```python
from build123d import *

# Parameters (mm, degrees)
SKETCH1_R           = 20
BOSS_EXTRUDE1_DEPTH = 5
SKETCH3_R           = 3
BOSS_EXTRUDE2_DEPTH = 11
CUT_EXTRUDE1_DEPTH  = 6


with BuildPart() as part:
    # Sketch1 → Boss-Extrude1 (new body)
    with BuildSketch(Plane.XY):
        Circle(SKETCH1_R)
    extrude(amount=BOSS_EXTRUDE1_DEPTH)

    # Sketch3 → Boss-Extrude2 (add)
    with BuildSketch(Plane.XY.offset(5)):
        with Locations((-15, 0)):
            Circle(SKETCH3_R)
    extrude(amount=BOSS_EXTRUDE2_DEPTH)

    # Sketch5 → Cut-Extrude1 (cut, through all)
    with BuildSketch(Plane.XY.offset(5)):
        with BuildLine():
            Line((5.656854249, 2), (7.5, 2))
            Line((7.5, 2), (7.5, -2))
            Line((7.5, -2), (5.656854249, -2))
            ThreePointArc((5.656854249, -2), (-6, 0), (5.656854249, 2))
        make_face()
    extrude(amount=-CUT_EXTRUDE1_DEPTH, mode=Mode.SUBTRACT)


solid = part.part
```
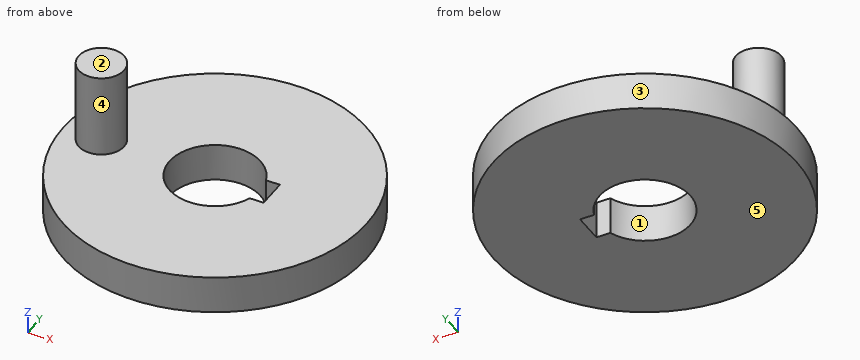
Check sheet for the modelled part. Datum: model origin and axes. Units: mm. Face numbers are marked on the shaded views. A direction names the side the tool comes from. Round coordinates to 2 decimals unless told otherwise and drop trailing zeros. Write each loop counter-clockwise with the first axis right and the second up, starting at its lowest first coordinate (ties: lowest second). Pieces come first, ordered by that corner, then holes. Notation, with made-up numbers: (53, 21) -> (65, 21) arc R14 cw to (65, 26) -> close; hole circle Ø2 at (-0.75, 32). An arc over 180 degrees is marked (long way). One line per question, with ' | ' between items. Start each with the question number.
1. Set-up check for the marked faces 4 and 5: record each of +Z, -Z, +X, -X, +Y, -Y from which the full face is reachable in a straight line by a thin tool's end or side.
2. Sectioned sample at D-D, the plane x = -15. Record the cut outline in (y, z).
3. Sectioned sample at C-C, the plane z = 1.5. Record the cut outline in (x, y).
4. Sectioned sample at B-B, the plane y = -1. Record the cut outline in (x, z), then the cut area to 3 significant figures.
5. Scan lines: line 1 along Y through (x, z) = (0, 1.9); line 2 along Z through (x, y) = (-2, -13.5); line 3 along Y through (x, z) = (4.5, 2). Record each from-to range of solid material in increasing order. Write a range as from..to.
6. Release check for a two-part mould opening along X. For the marked faces 1, 2 and 3 record: +X half, -X half, draft (parallel to the pull), parting line (faces both ways), or undercut.
7. Sectioned sample at A-A, the plane x = 0. Record the cut outline in (y, z).
8. Depth check by flat-ended pin: pin 1 (1 mm diameter, centred on x = -1, y = -10.5, fed in from +Z); pin 2 (8 mm diameter, centred on y = -11, z = 12.5, fed in from +X); pin 3 (6 mm diameter, centred on y = -14, z = 4.5, fed in from +X); pin 4 (1.5 mm diameter, centred on x = 7, z = 3, fed in from +Y). Enter the tip coordinate at first touch or a pass-through.
Taken from the geometry:
1) face 4: +Z | face 5: -Z, +X, -X, +Y, -Y
2) outline: (-13.23, 0) -> (13.23, 0) -> (13.23, 5) -> (3, 5) -> (3, 16) -> (-3, 16) -> (-3, 5) -> (-13.23, 5) -> close
3) outline: circle Ø40 at (0, 0); hole (5.66, -2) -> (7.5, -2) -> (7.5, 2) -> (5.66, 2) arc R6 ccw (long way) to start
4) outline: (-19.97, 0) -> (-5.92, 0) -> (-5.92, 5) -> (-12.17, 5) -> (-12.17, 16) -> (-17.83, 16) -> (-17.83, 5) -> (-19.97, 5) -> close; (7.5, 0) -> (19.97, 0) -> (19.97, 5) -> (7.5, 5) -> close | area: 195 mm^2
5) line 1: y = -20..-6, 6..20 | line 2: z = 0..5 | line 3: y = -19.49..-3.97, 3.97..19.49
6) face 1: undercut | face 2: draft | face 3: parting line
7) outline: (-20, 0) -> (-6, 0) -> (-6, 5) -> (-20, 5) -> close; (6, 0) -> (20, 0) -> (20, 5) -> (6, 5) -> close
8) pin 1: stops at z = 5 | pin 2: passes through | pin 3: stops at x = 16.7 | pin 4: stops at y = 19
